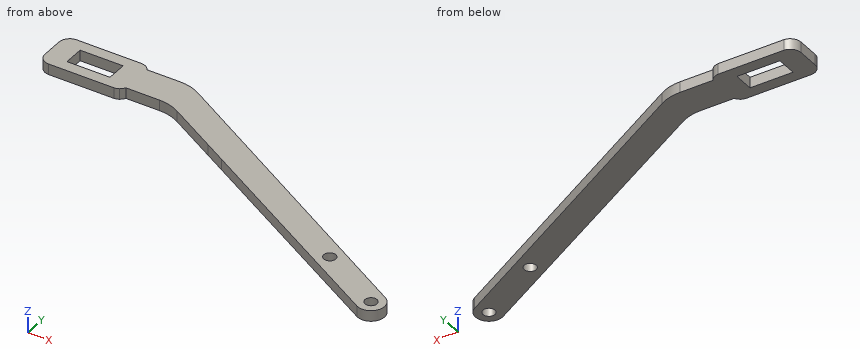
from build123d import *

# Parameters (mm, degrees)
SKETCH1_R                       = 1.7859375
SKETCH1_W                       = 12.7
SKETCH1_H                       = 5.9944
BOSS_EXTRUDE1_DEPTH             = 3.175
FILLET2_R                       = 12.7
F_9_64_0_14063_DIAMETER_HOLE1_D = 3.572002


with BuildPart() as part:
    # Sketch1 → Boss-Extrude1 (new body)
    with BuildSketch(Plane.XY):
        with BuildLine():
            Line((-25.595614794, 12.127914856), (-24.431663343, 13.29684081))
            Line((-24.431663343, 13.29684081), (-11.306294, 13.29684081))
            Line((-11.306294, 13.29684081), (6.117359384, 3.377856252))
            Line((6.117359384, 3.377856252), (12.411791243, -0.205454953))
            Line((12.411791243, -0.205454953), (75.625928444, -36.192170077))
            ThreePointArc((75.625928444, -36.192170077), (81.03522907, -34.712213349), (79.564057068, -29.300516931))
            Line((79.564057068, -29.300516931), (-11.306294, 22.82184081))
            Line((-11.306294, 22.82184081), (-24.431663343, 22.82184081))
            ThreePointArc((-24.431663343, 22.82184081), (-25.519216943, 23.940247646), (-27.007802046, 24.406853559))
            Line((-27.007802046, 24.406853559), (-46.413402046, 24.406853559))
            ThreePointArc((-46.413402046, 24.406853559), (-48.546190424, 23.416669154), (-49.415576549, 21.231853559))
            Line((-49.415576549, 21.231853559), (-49.415576549, 14.881853559))
            ThreePointArc((-49.415576549, 14.881853559), (-48.546190424, 12.697037963), (-46.413402046, 11.706853559))
            Line((-46.413402046, 11.706853559), (-27.007802046, 11.706853559))
            ThreePointArc((-27.007802046, 11.706853559), (-26.27698161, 11.834453561), (-25.595614794, 12.127914856))
        make_face()
        with Locations((77.589397954, -32.743146441)):
            Circle(SKETCH1_R, mode=Mode.SUBTRACT)
        with Locations((-36.710602046, 18.056853559)):
            Rectangle(SKETCH1_W, SKETCH1_H, mode=Mode.SUBTRACT)
    extrude(amount=BOSS_EXTRUDE1_DEPTH)

    # Fillet2
    fillet2_edges = [part.edges().sort_by_distance(p)[0] for p in [
        (-11.306294, 22.82184081, 1.5875),
        (-11.306294, 13.29684081, 1.5875),
    ]]
    fillet(fillet2_edges, radius=FILLET2_R)

    # 9/64 (0.14063) Diameter Hole1 (through all)
    with Locations(Plane.XY.offset(3.175)):
        with Locations((58.292743709, -21.716371758)):
            Hole(F_9_64_0_14063_DIAMETER_HOLE1_D / 2)


solid = part.part
The listing builds one solid part. Answer for the finished solid, in the listing's coordinates (mm). Coordinates: 2 decimals unless noted, no trailing zeros. Write each loop counter-clockwise with the first axis right and the second up, starting at its lowest first coordinate (ties: lowest second). Pieces come first, ordered by that corner, then holes. Notation, with made-up numbers: M 83,82.5 L 133,82.5 A8 ccw 133,93.5 Z; hole C 78,-9.5 d2. An arc over 180 degrees is marked long. Put each result on its own line as item: value. Start each with the question number.
1. A cutting plane is placed at B-B on z = 1.2. Write down the section's boundary in (x, y).
2. Consider line 1 (Y direction, x = -35.5, z = 2.3); line 2 (Y direction, x = -21.5, z = 2.8); line 3 (X direction, y = 19.5, z = 2.75). Determine where each line is inside the solid, lowest interval first. Write a range as from..to.
3. Flat-ended cylindrical pins translate along their axes: P1, Ø3, axis at x = 77.59, y = -32.74, coming from the -Z side; P2, Ø1.5, axis at x = 21.5, z = 2, coming from the +Y side; P3, Ø1.5, axis at y = 6.5, z = 3, coming from the +X side; P4, Ø1, axis at x = -18.5, z = 2, coming from the +Y side. Find the tip coordinate at first contact, or state that the pin passes through.
4. A cutting plane is placed at A-A on x = -35. Write down the section's boundary in (y, z) (3 decimals), then the cut area to 3 significant figures.
5. A cutting plane is placed at C-C on y = -28. Write down the section's boundary in (x, z) (3 decimals).
6. A cutting plane is placed at D-D on x = 66. Write down the section's boundary in (y, z) (3 decimals).
Resolved:
1. outline: M -49.42,14.88 A3.18 ccw -46.41,11.71 L -27.01,11.71 A3.18 ccw -25.6,12.13 L -24.43,13.3 L -14.67,13.3 A12.7 cw -8.38,11.63 L 75.63,-36.19 A3.97 ccw 79.56,-29.3 L -8.37,21.14 A12.7 ccw -14.69,22.82 L -24.43,22.82 A3.18 ccw -27.01,24.41 L -46.41,24.41 A3.18 ccw -49.42,21.23 Z; hole M -43.06,15.06 L -30.36,15.06 L -30.36,21.05 L -43.06,21.05 Z; hole C 58.29,-21.72 d3.57; hole C 77.59,-32.74 d3.57
2. line 1: y = 11.71..15.06, 21.05..24.41
2. line 2: y = 13.3..22.82
2. line 3: x = -49.42..-43.06, -30.36..-5.51
3. P1: passes through
3. P2: stops at y = 4.43
3. P3: stops at x = 18.46
3. P4: stops at y = 22.82
4. outline: M 11.707,0 L 15.06,0 L 15.06,3.175 L 11.707,3.175 Z; M 21.054,0 L 24.407,0 L 24.407,3.175 L 21.054,3.175 Z
4. area: 21.3 mm2
5. outline: M 61.236,0 L 77.297,0 L 77.297,3.175 L 61.236,3.175 Z
6. outline: M -30.712,0 L -21.52,0 L -21.52,3.175 L -30.712,3.175 Z
